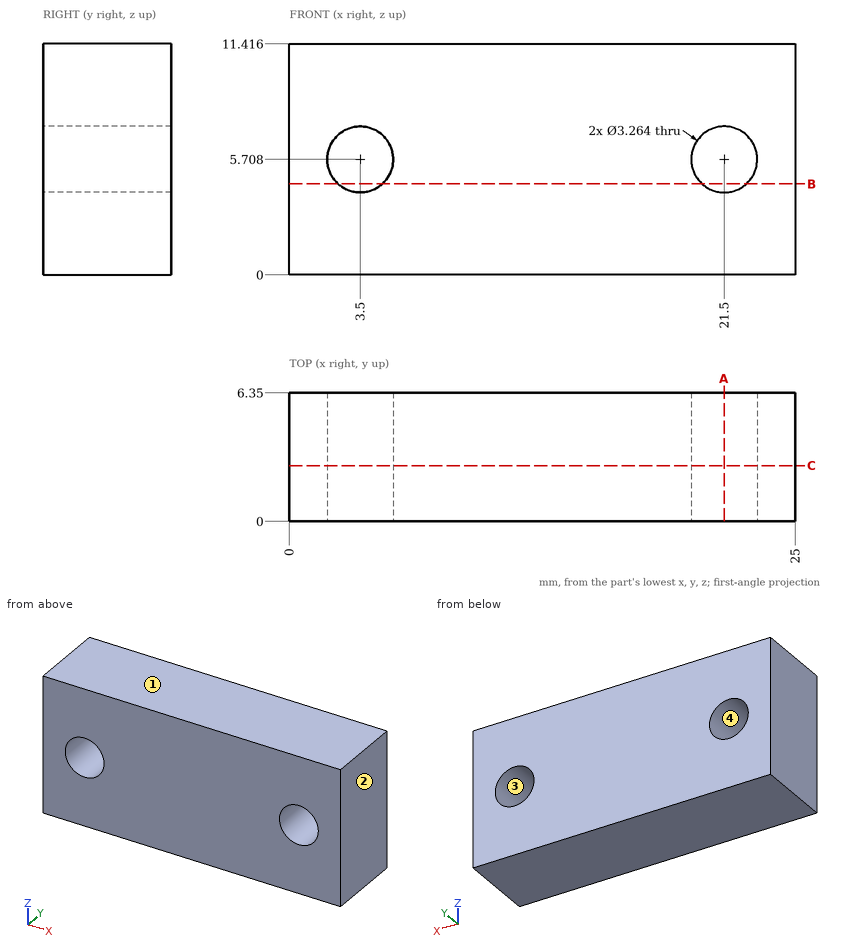
Source: three-view drawing plus pictorial views. Frame: mm from the lowest corner of the part. Give positions to 0.01 mm unless a question says otherwise; leave off trailing zeros. Order: outer loops, then holes, each group sorted by start corner. A loop starts at its lowest first (then second) coordinate and runs counter-clockwise, first axis right, second up. Notation, with made-up numbers: M -39,6.25 L -1,6.25 A19 cw -1,17.25 Z; hole C 56,-23.5 d3. An arc over 180 degrees is marked long. One line per question, with ' | ' between items.
1) Draft query along Z for the marked faces 1, 2, 3 and 4. Return one class per face: pulls with the +Z half, pulls with the -Z half, needs draft (parallel to the pull), parting line crosses it, or undercut.
Filled in:
face 1: pulls with the +Z half | face 2: needs draft | face 3: undercut | face 4: undercut
2) Section A-A on x = 21.5. Output: boundary loops of the cut face in (y, z), and give its area (3 significant figures).
Filled in:
outline: M 0,0 L 6.35,0 L 6.35,4.08 L 0,4.08 Z; M 0,7.34 L 6.35,7.34 L 6.35,11.42 L 0,11.42 Z | area: 51.8 mm2
3) Ray query, L1, parallel to X at y = 2.25, z = 5.75; L2, parallel to Z at x = 21.5, y = 3.5; L3, parallel to X at y = 3.25, z = 6.5. Return the intervals inside material, ascending.
Filled in:
L1: x = 0 to 1.87, 5.13 to 19.87, 23.13 to 25 | L2: z = 0 to 4.08, 7.34 to 11.42 | L3: x = 0 to 2.07, 4.93 to 20.07, 22.93 to 25
4) Contact query for a flat-ended pin moving along its axis: P1, Ø2.5, axis at x = 21.5, z = 5.708, coming from the +Y side. Output: stop coordinate, or through.
Filled in:
P1: passes through
5) Section C-C on y = 2.75. Output: boundary loops of the cut face in (x, z), and give its area (3 significant figures).
Filled in:
outline: M 0,0 L 25,0 L 25,11.42 L 0,11.42 Z; hole C 3.5,5.71 d3.26; hole C 21.5,5.71 d3.26 | area: 269 mm2
6) Section B-B on z = 4.5. Output: boundary loops of the cut face in (x, y).
Filled in:
outline: M 0,0 L 2.4,0 L 2.4,6.35 L 0,6.35 Z; M 4.6,0 L 20.4,0 L 20.4,6.35 L 4.6,6.35 Z; M 22.6,0 L 25,0 L 25,6.35 L 22.6,6.35 Z
